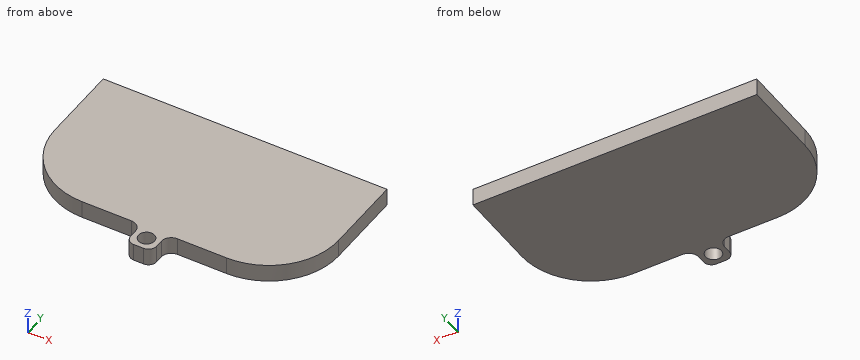
from build123d import *

# Parameters (mm, degrees)
BOSS_EXTRUDE1_DEPTH = 3.5
SKETCH2_R           = 1.6
BOSS_EXTRUDE2_DEPTH = 3.5
FILLET1_R           = 2


with BuildPart() as part:
    # Sketch1 → Boss-Extrude1 (new body)
    with BuildSketch(Plane.XY):
        with BuildLine():
            Line((-24.5, 0), (24.5, 0))
            Line((24.5, 0), (28.5, 0))
            Line((28.5, 0), (28.5, -16))
            ThreePointArc((28.5, -16), (24.399494937, -25.899494937), (14.5, -30))
            Line((14.5, -30), (-14.5, -30))
            ThreePointArc((-14.5, -30), (-24.399494937, -25.899494937), (-28.5, -16))
            Line((-28.5, -16), (-28.5, 0))
            Line((-28.5, 0), (-24.5, 0))
        make_face()
    extrude(amount=BOSS_EXTRUDE1_DEPTH)

    # Sketch2 → Boss-Extrude2 (add)
    with BuildSketch(Plane.XY.offset(3.5)):
        with BuildLine():
            Line((2.6, -30), (-2.6, -30))
            Line((-2.6, -30), (-2.6, -33.6))
            ThreePointArc((-2.6, -33.6), (-2.13137085, -34.73137085), (-1, -35.2))
            Line((-1, -35.2), (1, -35.2))
            ThreePointArc((1, -35.2), (2.13137085, -34.73137085), (2.6, -33.6))
            Line((2.6, -33.6), (2.6, -30))
        make_face()
        with Locations((0, -32.6)):
            Circle(SKETCH2_R, mode=Mode.SUBTRACT)
    extrude(amount=-BOSS_EXTRUDE2_DEPTH)

    # Fillet1
    fillet1_edges = [part.edges().sort_by_distance(p)[0] for p in [
        (2.6, -30, 1.75),
        (-2.6, -30, 1.75),
    ]]
    fillet(fillet1_edges, radius=FILLET1_R)


solid = part.part
Work out the finished part from the listing and answer in its coordinate system (mm). Give positions to 0.01 mm unless a question says otherwise; leave off trailing zeros. Order: outer loops, then holes, each group sorted by start corner. A loop starts at its lowest first (then second) coordinate and runs counter-clockwise, first axis right, second up. Notation, with made-up numbers: (-11, 49.5) -> (47, 49.5) arc R15 ccw to (47, 65.5) -> close; hole circle Ø8 at (60, 20.5). An arc over 180 degrees is marked (long way). Answer as a JSON object with one key per item and string values. Group by question number.
1. Section C-C on z = 2.6 is taken. Determine the outline of the cut face in (x, y), plus the area to 3 significant figures.
2. Section A-A on y = -32.6 is taken. Determine the outline of the cut face in (x, z), plus the area to 3 significant figures.
3. Section B-B on x = 0 is taken. Determine the outline of the cut face in (y, z), plus the area to 3 significant figures.
4. Section D-D on x = 12.5 is taken. Determine the outline of the cut face in (y, z), plus the area to 3 significant figures.
5. Flat-ended cylindrical pins translate along their axes: pin 1 Ø1.3 at (y, z) = (-33, 2.5) entering from -X; pin 2 Ø2 at (x, z) = (-4.5, 3) entering from -Y; pin 3 Ø1.3 at (y, z) = (-32.5, 2.5) entering from +X. Find the tip coordinate at first contact, or state that the pin passes through.
6. Consider line 1 along Y through (x, z) = (0, 1.8); line 2 along Y through (x, z) = (9, 2.95); line 3 along X through (y, z) = (-32, 3.35). Determine where each line is inside the solid, lowest interval first. Write a range as [from, to].
Result sheet:
{
 "1": {"outline": "(-28.5, -16) arc R14 ccw to (-14.5, -30) -> (-4.6, -30) arc R2 cw to (-2.6, -32) -> (-2.6, -33.6) arc R1.6 ccw to (-1, -35.2) -> (1, -35.2) arc R1.6 ccw to (2.6, -33.6) -> (2.6, -32) arc R2 cw to (4.6, -30) -> (14.5, -30) arc R14 ccw to (28.5, -16) -> (28.5, 0) -> (-28.5, 0) -> close; hole circle Ø3.2 at (0, -32.6)", "area": "1,650 mm^2"},
 "2": {"outline": "(-2.6, 0) -> (-1.6, 0) -> (-1.6, 3.5) -> (-2.6, 3.5) -> close; (1.6, 0) -> (2.6, 0) -> (2.6, 3.5) -> (1.6, 3.5) -> close", "area": "7.00 mm^2"},
 "3": {"outline": "(-35.2, 0) -> (-34.2, 0) -> (-34.2, 3.5) -> (-35.2, 3.5) -> close; (-31, 0) -> (0, 0) -> (0, 3.5) -> (-31, 3.5) -> close", "area": "112 mm^2"},
 "4": {"outline": "(-30, 0) -> (0, 0) -> (0, 3.5) -> (-30, 3.5) -> close", "area": "105 mm^2"},
 "5": {"pin 1": "stops at x = -2.6", "pin 2": "stops at y = -30.33", "pin 3": "stops at x = 2.61"},
 "6": {"line 1": "y = [-35.2, -34.2], [-31, 0]", "line 2": "y = [-30, 0]", "line 3": "x = [-2.6, -1.48], [1.48, 2.6]"}
}
